Check sheet for the modelled part. Datum: model origin and axes. Units: mm. A direction names the side the tool comes from. Give positions to 0.01 mm unless a question says otherwise; leave off trailing zeros. Order: outer loops, then holes, each group sorted by start corner. A loop starts at its lowest first (then second) coordinate and runs counter-clockwise, first axis right, second up.
```python
from build123d import *

# Parameters (mm, degrees)
EXTRUDE_THIN1_DEPTH = 5


with BuildPart() as part:
    # Sketch2 → Extrude-Thin1 (new body)
    with BuildSketch(Plane.XY):
        with BuildLine():
            Line((14.887131394, 82.636077838), (4.256350187, -7.49933382))
            ThreePointArc((4.256350187, -7.49933382), (-10.506003475, -18.916342962), (-21.634589327, -3.93536301))
            Line((-21.634589327, -3.93536301), (3.361011475, 154.797495405))
            ThreePointArc((3.361011475, 154.797495405), (35.58717678, 173.770376713), (47.983576242, 138.488295769))
            Line((47.983576242, 138.488295769), (15.851718131, 85.44288319))
            ThreePointArc((15.851718131, 85.44288319), (15.218957799, 84.091189991), (14.887131394, 82.636077838))
        make_face()
        with BuildLine():
            Line((9.921548726, 83.221730268), (-0.709232481, -6.91368139))
            ThreePointArc((-0.709232481, -6.91368139), (-9.824166991, -13.963051227), (-16.695451446, -4.71312711))
            Line((-16.695451446, -4.71312711), (8.300149356, 154.019731305))
            ThreePointArc((8.300149356, 154.019731305), (33.870766271, 169.074214987), (43.706984101, 141.078809165))
            Line((43.706984101, 141.078809165), (11.575125989, 88.033396586))
            ThreePointArc((11.575125989, 88.033396586), (10.490393993, 85.716208245), (9.921548726, 83.221730268))
        make_face(mode=Mode.SUBTRACT)
    extrude(amount=-EXTRUDE_THIN1_DEPTH)


solid = part.part
```
(1) Cross-section at B-B on y = 151.5. Enter the section's corners in (x, z).
Response values:
outline: (2.84, -5) - (7.9, -5) - (7.9, 0) - (2.84, 0) - close; (46.48, -5) - (51.48, -5) - (51.48, 0) - (46.48, 0) - close
(2) Gauge pin test, flat end, axial feed: pin 1 Ø1 at (y, z) = (24, -3.5) entering from -X. Record the tip position at first contact, or that the pin passes through.
Response values:
pin 1: stops at x = -17.31
(3) Cross-section at A-A on x = -5.5. Enter the section's corners in (y, z).
Response values:
outline: (-18.63, -5) - (-13.37, -5) - (-13.37, 0) - (-18.63, 0) - close; (66.38, -5) - (98.53, -5) - (98.53, 0) - (66.38, 0) - close
(4) Release check for a two-part mould opening along Y. For faces 1 (the face through (33.423, 169.232, -2.465)), 2 (the face through (12, 86, -5)), 3 (the face through (9.646, 38.199, -2.465)), 4 (the face through (27.866, 114.927, -2.465)) record: released by +Y, released by -Y, zero draft, split by the parting line, or undercut.
Response values:
face 1: undercut
face 2: zero draft
face 3: released by -Y
face 4: undercut
(5) Set-up check for faces 5 (the face through (12, 86, 0)), 6 (the face through (-4.373, 73.542, -2.465)): record each of +Z, -Z, +X, -X, +Y, -Y from which the full face is reachable in a straight line by a thin tool's end or side.
Response values:
face 5: +Z, +X, -X, +Y, -Y
face 6: +Z, -Z
(6) Material ranges on L1, parallel to Y at x = 41, z = -3.5; L2, parallel to X at y = 106, z = -1.4; L3, parallel to Y at x = 22, z = -3.7, recorded low to high.
Response values:
L1: y = 126.96 to 136.61, 164.47 to 170.98
L2: x = -4.32 to 0.74, 22.46 to 28.3
L3: y = 95.59 to 105.24, 169.5 to 174.66
(7) Cross-section at C-C on z = -2.2. Enter the section's corners in (x, y).
Response values:
outline: (-21.63, -3.94) arc R13.07 ccw (long way) to (4.26, -7.5) - (14.89, 82.64) arc R7 cw to (15.85, 85.44) - (47.98, 138.49) arc R24.21 ccw (long way) to (3.36, 154.8) - close; hole (-16.7, -4.71) arc R8.07 ccw (long way) to (-0.71, -6.91) - (9.92, 83.22) arc R12 cw to (11.58, 88.03) - (43.71, 141.08) arc R19.21 ccw (long way) to (8.3, 154.02) - close
